Input: part model. Units: mm. Frame: model coordinates. A direction names the side the tool comes from. Round coordinates to 2 decimals unless told otherwise and drop trailing zeros. Loops run counter-clockwise (first coordinate to the right, second up) from the corner with the lowest first, then second, coordinate; pieces in that order, holes last.
(1) Access query for faces 1 (the face through (-1, 13, 5)), 2 (the face through (10, 0, 2)). Directions: +Z, -Z, +X, -X, +Y, -Y. A direction counts if a zero-diameter tool reaches every point of the face in a straight line with its end or side. Return the directions, or none.
(2) Draft query along X for faces 3 (the face through (-1, 13, 0)), 4 (the face through (45.237, 11.35, 2.465)), 5 (the face through (3, 8.32, 2)), 6 (the face through (-43.99, -10.12, 2.46)). Return one class per face: released by +X, released by -X, zero draft, split by the parting line, or undercut.
(3) Cut plane C-C, the plane y = 42. Output: boundary loops of the cut face in (x, z), and give its area (3 significant figures).
(4) First-contact query: pin 1 Ø1.3 at (x, z) = (-19.5, 3) entering from +Y; pin 2 Ø1.5 at (x, z) = (-33.5, 1.5) entering from +Y; pin 3 Ø2 at (x, z) = (45.5, 1.5) entering from -Y; pin 4 Ø5 at (x, y) = (3, -18) entering from -Z. Flat tips, straight axial feed; report the tip coordinate or a pass-through.
(5) Line query: line 1 (Y direction, x = -46, z = 3.45); line 2 (X direction, y = 21.5, z = 2.15); line 3 (Y direction, x = -8, z = 1.35). Output: solid intervals per line, ascending.
(6) Cut plane A-A, the plane z = 1.3. Give the number of separate pieces and of enclosed holes in the cut face, and give its area (3 significant figures).
(7) Cut plane B-B, the plane y = -18. Output: boundary loops of the cut face in (x, z).
from build123d import *

# Parameters (mm, degrees)
F1_DEPTH = 5


with BuildPart() as f1:
    # F0 (on Top) → F1 (new body)
    with BuildSketch(Plane.XY):
        with BuildLine():
            ThreePointArc((39.9847812951, -13.5503625497), (43.9367876921, -10.1710657097), (47.5637614727, -6.445067469))
            ThreePointArc((47.5637614727, -6.445067469), (57.7574296409, 22.7274453414), (44.4848015904, 50.6341420114))
            ThreePointArc((44.4848015904, 50.6341420114), (21.3589499339, 58.3817468835), (0, 46.6078072786))
            ThreePointArc((0, 46.6078072786), (-21.3589499339, 58.3817468835), (-44.4848015904, 50.6341420114))
            ThreePointArc((-44.4848015904, 50.6341420114), (-57.7574296409, 22.7274453414), (-47.5637614727, -6.445067469))
            ThreePointArc((-47.5637614727, -6.445067469), (-43.9367876921, -10.1710657097), (-39.9847812951, -13.5503625497))
            ThreePointArc((-39.9847812951, -13.5503625497), (-17.6817313741, -34.786119341), (0, -60))
            ThreePointArc((0, -60), (17.6817313741, -34.786119341), (39.9847812951, -13.5503625497))
        make_face()
        with BuildLine():
            add(Edge.make_bspline(
                [(-38.2190007028, 6.1661579287), (-37.656258132, 5.2612678749), (-37.656258132, 4.0517465095)],
                knots=[0, 0, 0, 1, 1, 1], degree=2))
            add(Edge.make_bspline(
                [(-37.656258132, 4.0517465095), (-37.656258132, 2.0919017164), (-39.0443564732, 0.9514101063)],
                knots=[0, 0, 0, 1, 1, 1], degree=2))
            add(Edge.make_bspline(
                [(-39.0443564732, 0.9514101063), (-40.4324548144, -0.1890815038), (-42.8034768459, -0.1890815038)],
                knots=[0, 0, 0, 1, 1, 1], degree=2))
            add(Edge.make_bspline(
                [(-42.8034768459, -0.1890815038), (-44.8773708, -0.1890815038), (-46.143916746, 0.6572833227)],
                knots=[0, 0, 0, 1, 1, 1], degree=2))
            Line((-46.143916746, 0.6572833227), (-46.143916746, 3.226390739))
            add(Edge.make_bspline(
                [(-46.143916746, 3.226390739), (-44.3341366384, 2.2149547585), (-42.7854690837, 2.2149547585)],
                knots=[0, 0, 0, 1, 1, 1], degree=2))
            add(Edge.make_bspline(
                [(-42.7854690837, 2.2149547585), (-41.7350162849, 2.2149547585), (-41.1437614239, 2.6126261752)],
                knots=[0, 0, 0, 1, 1, 1], degree=2))
            add(Edge.make_bspline(
                [(-41.1437614239, 2.6126261752), (-40.5525065629, 3.0102975919), (-40.5525065629, 3.7035964391)],
                knots=[0, 0, 0, 1, 1, 1], degree=2))
            add(Edge.make_bspline(
                [(-40.5525065629, 3.7035964391), (-40.5525065629, 4.10877109), (-40.6800615456, 4.4134024016)],
                knots=[0, 0, 0, 1, 1, 1], degree=2))
            add(Edge.make_bspline(
                [(-40.6800615456, 4.4134024016), (-40.8076165283, 4.7180337133), (-41.0417174377, 4.980646913)],
                knots=[0, 0, 0, 1, 1, 1], degree=2))
            add(Edge.make_bspline(
                [(-41.0417174377, 4.980646913), (-41.2758183472, 5.2432601127), (-42.2032181038, 5.9365589599)],
                knots=[0, 0, 0, 1, 1, 1], degree=2))
            add(Edge.make_bspline(
                [(-42.2032181038, 5.9365589599), (-43.4997769868, 6.8669600102), (-44.0250033862, 7.7763520045)],
                knots=[0, 0, 0, 1, 1, 1], degree=2))
            add(Edge.make_bspline(
                [(-44.0250033862, 7.7763520045), (-44.5502297856, 8.6857439989), (-44.5502297856, 9.7361967977)],
                knots=[0, 0, 0, 1, 1, 1], degree=2))
            add(Edge.make_bspline(
                [(-44.5502297856, 9.7361967977), (-44.5502297856, 10.9457181631), (-43.9679788057, 11.8971282694)],
                knots=[0, 0, 0, 1, 1, 1], degree=2))
            add(Edge.make_bspline(
                [(-43.9679788057, 11.8971282694), (-43.3857278258, 12.8485383757), (-42.3112646774, 13.3782667156)],
                knots=[0, 0, 0, 1, 1, 1], degree=2))
            add(Edge.make_bspline(
                [(-42.3112646774, 13.3782667156), (-41.2368015289, 13.9079950556), (-39.8411999534, 13.9079950556)],
                knots=[0, 0, 0, 1, 1, 1], degree=2))
            add(Edge.make_bspline(
                [(-39.8411999534, 13.9079950556), (-37.8063228175, 13.9079950556), (-36.1165944584, 12.980595299)],
                knots=[0, 0, 0, 1, 1, 1], degree=2))
            Line((-36.1165944584, 12.980595299), (-37.1400356138, 10.7956534775))
            add(Edge.make_bspline(
                [(-37.1400356138, 10.7956534775), (-38.6016656509, 11.4889523247), (-39.8411999534, 11.4889523247)],
                knots=[0, 0, 0, 1, 1, 1], degree=2))
            add(Edge.make_bspline(
                [(-39.8411999534, 11.4889523247), (-40.6185350245, 11.4889523247), (-41.1152491336, 11.0672705584)],
                knots=[0, 0, 0, 1, 1, 1], degree=2))
            add(Edge.make_bspline(
                [(-41.1152491336, 11.0672705584), (-41.6119632428, 10.645588792), (-41.6119632428, 9.9522899448)],
                knots=[0, 0, 0, 1, 1, 1], degree=2))
            add(Edge.make_bspline(
                [(-41.6119632428, 9.9522899448), (-41.6119632428, 9.3790428461), (-41.3028299906, 8.9528591391)],
                knots=[0, 0, 0, 1, 1, 1], degree=2))
            add(Edge.make_bspline(
                [(-41.3028299906, 8.9528591391), (-40.9936967383, 8.5266754322), (-39.9162322962, 7.8213714102)],
                knots=[0, 0, 0, 1, 1, 1], degree=2))
            add(Edge.make_bspline(
                [(-39.9162322962, 7.8213714102), (-38.7817432735, 7.0710479825), (-38.2190007028, 6.1661579287)],
                knots=[0, 0, 0, 1, 1, 1], degree=2))
        make_face(mode=Mode.SUBTRACT)
        Polygon((-27.2237611935, 2.4010349686), (-27.7219759494, 0), (-36.9239424666, 0), (-36.566788515, 1.8848124503), (-29.2796473853, 11.3118759958), (-34.3728428124, 11.3118759958), (-33.8746280565, 13.7129109644), (-25.0958439525, 13.7129109644), (-25.4800095475, 11.8190946329), (-32.8151713766, 2.4010349686), align=None, mode=Mode.SUBTRACT)
        Polygon((-17.3855204096, 2.4010349686), (-17.8927390468, 0), (-25.5550418903, 0), (-22.6587934594, 13.7129109644), (-14.984485441, 13.7129109644), (-15.4917040782, 11.3298837581), (-20.2937740153, 11.3298837581), (-20.9240456946, 8.3195861662), (-16.4491167719, 8.3195861662), (-16.9653392901, 5.9365589599), (-21.4372669191, 5.9365589599), (-22.1875903468, 2.4010349686), align=None, mode=Mode.SUBTRACT)
        with BuildLine():
            Line((-10.0503585806, 5.2612678749), (-11.166839841, 5.2612678749))
            Line((-11.166839841, 5.2612678749), (-12.2833211014, 0))
            Line((-12.2833211014, 0), (-15.1435540077, 0))
            Line((-15.1435540077, 0), (-12.2473055768, 13.7129109644))
            Line((-12.2473055768, 13.7129109644), (-8.8798540334, 13.7129109644))
            add(Edge.make_bspline(
                [(-8.8798540334, 13.7129109644), (-6.6558953937, 13.7129109644), (-5.5394141333, 12.7554982707)],
                knots=[0, 0, 0, 1, 1, 1], degree=2))
            add(Edge.make_bspline(
                [(-5.5394141333, 12.7554982707), (-4.4229328729, 11.7980855769), (-4.4229328729, 9.9522899448)],
                knots=[0, 0, 0, 1, 1, 1], degree=2))
            add(Edge.make_bspline(
                [(-4.4229328729, 9.9522899448), (-4.4229328729, 8.4696508517), (-5.2017685909, 7.4056922313)],
                knots=[0, 0, 0, 1, 1, 1], degree=2))
            add(Edge.make_bspline(
                [(-5.2017685909, 7.4056922313), (-5.9806043088, 6.3417336108), (-7.4452356397, 5.8255110926)],
                knots=[0, 0, 0, 1, 1, 1], degree=2))
            Line((-7.4452356397, 5.8255110926), (-4.9961799717, 0))
            Line((-4.9961799717, 0), (-8.1115228434, 0))
            Line((-8.1115228434, 0), (-10.0503585806, 5.2612678749))
        make_face(mode=Mode.SUBTRACT)
        Polygon((4.7220090637, 2.4010349686), (4.2147904266, 0), (-3.4475124169, 0), (-0.5512639861, 13.7129109644), (7.1230440323, 13.7129109644), (6.6158253952, 11.3298837581), (1.813755458, 11.3298837581), (1.1834837787, 8.3195861662), (5.6584127015, 8.3195861662), (5.1421901832, 5.9365589599), (0.6702625542, 5.9365589599), (-0.0800608735, 2.4010349686), align=None, mode=Mode.SUBTRACT)
        Polygon((14.2030958959, 11.2938682335), (11.8200686896, 0), (8.9598357833, 0), (11.3428629896, 11.2938682335), (8.0414399078, 11.2938682335), (8.557662426, 13.7129109644), (18.0297453771, 13.7129109644), (17.5135228589, 11.2938682335), align=None, mode=Mode.SUBTRACT)
        Polygon((24.8216730445, 0), (17.159370201, 0), (20.0556186319, 13.7129109644), (22.9278567131, 13.7129109644), (20.5268217445, 2.4010349686), (25.3288916817, 2.4010349686), align=None, mode=Mode.SUBTRACT)
        Polygon((35.2811816265, 2.4010349686), (34.7739629894, 0), (27.1116601458, 0), (30.0079085767, 13.7129109644), (37.6822165951, 13.7129109644), (37.174997958, 11.3298837581), (32.3729280208, 11.3298837581), (31.7426563415, 8.3195861662), (36.2175852642, 8.3195861662), (35.701362746, 5.9365589599), (31.229435117, 5.9365589599), (30.4791116893, 2.4010349686), align=None, mode=Mode.SUBTRACT)
        Polygon((44.9963693682, 7.1460803253), (47.7275466449, 0), (44.5551791927, 0), (42.5773266373, 5.5523933649), (41.4038207964, 4.8951100422), (40.3833809348, 0), (37.5231480284, 0), (40.4193964593, 13.7129109644), (43.2916345405, 13.7129109644), (41.8660200279, 7.128072563), (43.3456578273, 9.0519018316), (47.1813111896, 13.7129109644), (50.569771789, 13.7129109644), align=None, mode=Mode.SUBTRACT)
    extrude(amount=F1_DEPTH)


solid = f1.part
Reported:
1. face 1: +Z, +X, -X, +Y, -Y
1. face 2: +Z, -Z
2. face 3: zero draft
2. face 4: undercut
2. face 5: undercut
2. face 6: released by -X
3. outline: (-51.69, 0) - (51.69, 0) - (51.69, 5) - (-51.69, 5) - close
3. area: 517 mm2
4. pin 1: stops at y = 58.25
4. pin 2: stops at y = 57.24
4. pin 3: stops at y = -9.64
4. pin 4: stops at z = 0
5. line 1: y = -8.14 to 0.57, 3.15 to 49.19
5. line 2: x = -57.81 to 57.81
5. line 3: y = -47.26 to 0, 13.67 to 53.89
6. separate pieces: 1
6. enclosed holes: 9
6. area: 8,190 mm2
7. outline: (-34.53, 0) - (34.53, 0) - (34.53, 5) - (-34.53, 5) - close
